Design review of the part built by this model. Coordinates are the model's own, in mm. Coordinates: 2 decimals unless noted, no trailing zeros. Write each loop counter-clockwise with the first axis right and the second up, starting at its lowest first coordinate (ties: lowest second). Pieces come first, ordered by that corner, then holes. Notation, with made-up numbers: (-3, 67) - (43, 67) arc R22 ccw to (43, 98) - close; hole circle Ø9 at (57.25, 23). An arc over 180 degrees is marked (long way). Use a Markdown table: item, result.
from build123d import *

# Parameters (mm, degrees)
F0_R     = 16.65
F0_R_2   = 12.65
F1_DEPTH = 20
F2_DEPTH = 4
F3_SIZE  = 2
F4_R     = 1.99999


# Not quite as in the source:
# - a fillet or chamfer is up to 0.001 mm smaller than in the source, because OpenCascade refuses the exact size


with BuildPart() as f1:
    # F0 (on Top) → F1 (new body)
    with BuildSketch(Plane.XY):
        Circle(F0_R)
        Circle(F0_R_2, mode=Mode.SUBTRACT)
    extrude(amount=F1_DEPTH)

    # F0 (on Top) → F2 (join)
    with BuildSketch(Plane.XY):
        Circle(F0_R)
        Circle(F0_R_2, mode=Mode.SUBTRACT)
        Circle(F0_R_2)
    extrude(amount=-F2_DEPTH)

    # F3
    f3_edges = [f1.edges().sort_by_distance(p)[0] for p in [
        (-16.65, 0, -4),
    ]]
    chamfer(f3_edges, length=F3_SIZE)

    # F4 (radius 2 in the source; OpenCascade refuses exactly that, so slightly less here)
    f4_edges = [f1.edges().sort_by_distance(p)[0] for p in [
        (-12.65, 0, 20),
        (-16.65, 0, 20),
    ]]
    fillet(f4_edges, radius=F4_R)


solid = f1.part
(1) For pin 1 (1.5 mm diameter, centred on x = 2, y = 7, fed in from +Z); pin 2 (1.5 mm diameter, centred on x = -6.5, z = 13.5, fed in from -Y); pin 3 (6 mm diameter, centred on x = 1.5, z = 1.5, fed in from +Y); pin 4 (4 mm diameter, centred on x = 5, z = -1, fed in from +Y), all flat-tipped, find the tip position at first contact; note any pin that passes through.
Determined:
| item | result |
|---|---|
| pin 1 | z = 0 |
| pin 2 | y = -15.63 |
| pin 3 | y = 16.65 |
| pin 4 | y = 16.38 |
(2) Draft analysis for pull direction X (two halves, no side actions). For faces 1 (the flat face through (0, 0, 0)), 2 (the cylindrical face through (7.683, -14.771, 8.14)), 3 (the flat face through (0, 0, -4)), 4 (the cylindrical face through (-2.74, -12.35, 8.87)), state which applies: +X half, -X half, draft (parallel to the pull), parting line (faces both ways), or undercut.
Determined:
| item | result |
|---|---|
| face 1 | undercut |
| face 2 | parting line |
| face 3 | draft |
| face 4 | undercut |
(3) Take a section at C-C on z = 7.25. Write out the cut boundary in (x, y), and give its area (3 significant figures).
Determined:
| item | result |
|---|---|
| outline | circle Ø33.3 at (0, 0); hole circle Ø25.3 at (0, 0) |
| area | 368 mm2 |
(4) For L1, parallel to X at y = 0.5, z = 1.25; L2, parallel to Y at x = 0, z = 10.5; L3, parallel to Z at x = -6, y = -8, list the stretches that pass through material, from the lowest coordinate up. Write a range as from..to.
Determined:
| item | result |
|---|---|
| L1 | -16.64..-12.64, 12.64..16.64 |
| L2 | -16.65..-12.65, 12.65..16.65 |
| L3 | -4..0 |
